Read the model definition and answer for the solid it produces. Units are mm, in the model's axes. A direction names the side the tool comes from. Coordinates: 2 decimals unless noted, no trailing zeros. Write each loop counter-clockwise with the first axis right and the second up, starting at its lowest first coordinate (ties: lowest second). Pieces come first, ordered by that corner, then holes.
Item 1: Section C-C (y = 10) is taken. Give the vertices of the cut face in (x, z) (3 decimals).
Item 2: Section B-B (x = 35) is taken. Give the vertices of the cut face in (y, z), then the cut area to 3 significant figures.
Item 3: A tool of negligible diameter and unlimited length cuts with its end or side. For faces 1 (the face through (-38.028, 7.919, 8.452)), 2 (the face through (36, 7, 30)), 3 (the face through (-37.5, 6.6, -0.1)), 4 (the face through (13.155, 6.409, -31.352)), from which of +Z, -Z, +X, -X, +Y, -Y can it reach the whole face along a straight path? Write none if from no direction.
Item 4: Determine the mould class of faces 5 (the face through (-36, 7, 30)), 6 (the face through (-9, 13, -33)), 7 (the face through (-31.352, 6.409, -13.155)) for opening direction Y: released by +Y, released by -Y, zero draft, split by the parting line, or undercut.
Item 5: Section D-D (z = -35) is taken. Give the vertices of the cut face in (x, y), then the cut area to 3 significant figures.
Item 6: Each of these flat-tipped pins is pushed along its axis until it touches: P1, Ø1.3, axis at y = 5.5, z = 30, coming from the -X side; P2, Ø3.5, axis at y = 6.5, z = 10, coming from the +X side; P3, Ø5, axis at y = 8, z = -23, coming from the +X side. Where does it stop, or does it pass through?
Item 7: Section A-A (z = 10) is taken. Give the vertices of the cut face in (x, y).
Item 8: Straight lines are drawn through the part: probe 1 along X at (y, z) = (10.5, 6.5); probe 2 along Y at (x, z) = (-37, 10); probe 3 along X at (y, z) = (7.75, 0). For each, find the intervals that lie inside material, in ascending order.
from build123d import *

# Parameters (mm, degrees)
SKETCH_1_R          = 34
EXTRUDE_1_DEPTH     = 13
SKETCH_2_R          = 2.5
CUT_EXTRUDE_1_DEPTH = 59.043087444
SKETCH_3_W          = 68
SKETCH_3_H          = 40
CUT_EXTRUDE_2_DEPTH = 59.043087444
SKETCH_4_R          = 2.1
CUT_EXTRUDE_3_DEPTH = 4


with BuildPart() as part:
    # 草图1 → 凸台-拉伸1 (new body)
    with BuildSketch(Plane(origin=(0, 0, 0), x_dir=(1, 0, 0), z_dir=(0, 1, 0))):
        with BuildLine():
            Line((-40, 0), (-40, -40))
            Line((-40, -40), (40, -40))
            Line((40, -40), (40, 0))
            ThreePointArc((40, 0), (0, 40), (-40, 0))
        make_face()
        with Locations(Location((0, 0, 0), (0, 0, 90))):
            Circle(SKETCH_1_R, mode=Mode.SUBTRACT)
    extrude(amount=EXTRUDE_1_DEPTH)

    # 草图2 → 切除-拉伸1 (cut, through all)
    with BuildSketch(Plane(origin=(0, 13, 0), x_dir=(1, 0, 0), z_dir=(0, 1, 0))):
        with Locations((0, 35)):
            Circle(SKETCH_2_R)
        with Locations((24.748737342, 24.748737342)):
            Circle(SKETCH_2_R)
        with Locations((35, 0)):
            Circle(SKETCH_2_R)
        with Locations((24.748737342, -24.748737342)):
            Circle(SKETCH_2_R)
        with Locations((0, -35)):
            Circle(SKETCH_2_R)
        with Locations((-24.748737342, -24.748737342)):
            Circle(SKETCH_2_R)
        with Locations((-35, 0)):
            Circle(SKETCH_2_R)
        with Locations((-24.748737342, 24.748737342)):
            Circle(SKETCH_2_R)
    extrude(amount=-CUT_EXTRUDE_1_DEPTH, mode=Mode.SUBTRACT)

    # 草图3 → 切除-拉伸2 (cut, through all)
    with BuildSketch(Plane(origin=(0, 13, 0), x_dir=(1, 0, 0), z_dir=(0, 1, 0))):
        with Locations((0, -20)):
            Rectangle(SKETCH_3_W, SKETCH_3_H)
    extrude(amount=-CUT_EXTRUDE_2_DEPTH, mode=Mode.SUBTRACT)

    # 草图4 → 切除-拉伸3 (cut)
    with BuildSketch(Plane.ZY.offset(40)):
        with Locations((10, 6.5)):
            Circle(SKETCH_4_R)
        with Locations((30, 6.5)):
            Circle(SKETCH_4_R)
    cut_extrude_3 = extrude(amount=-CUT_EXTRUDE_3_DEPTH, mode=Mode.SUBTRACT)

    # 镜向1: 切除-拉伸3 across plane
    add(cut_extrude_3.mirror(Plane.ZY), mode=Mode.SUBTRACT)


solid = part.part
Established:
1. outline: (-40, 0) arc R40 ccw to (40, 0) - (40, 40) - (34, 40) - (34, 2.291) arc R2.5 cw (long way) to (33.925, -2.257) arc R34 cw to (25.585, -22.393) arc R2.5 cw (long way) to (22.393, -25.585) arc R34 cw to (2.257, -33.925) arc R2.5 cw (long way) to (-2.257, -33.925) arc R34 cw to (-22.393, -25.585) arc R2.5 cw (long way) to (-25.585, -22.393) arc R34 cw to (-33.925, -2.257) arc R2.5 cw (long way) to (-34, 2.291) - (-34, 40) - (-40, 40) - close
2. outline: (0, -19.36) - (13, -19.36) - (13, -2.5) - (0, -2.5) - close; (0, 2.5) - (13, 2.5) - (13, 40) - (0, 40) - close
2. area: 707 mm2
3. face 1: -X
3. face 2: +X
3. face 3: +Y, -Y
3. face 4: +Z, +Y, -Y
4. face 5: undercut
4. face 6: released by +Y
4. face 7: zero draft
5. outline: (-19.36, 0) - (-2.5, 0) - (-2.5, 13) - (-19.36, 13) - close; (2.5, 0) - (19.36, 0) - (19.36, 13) - (2.5, 13) - close
5. area: 438 mm2
6. P1: stops at x = -36
6. P2: stops at x = 36
6. P3: stops at x = 34.35
7. outline: (-40, 0) - (-34, 0) - (-34, 13) - (-40, 13) - (-40, 8.6) - (-36, 8.6) - (-36, 4.4) - (-40, 4.4) - close; (34, 0) - (40, 0) - (40, 4.4) - (36, 4.4) - (36, 8.6) - (40, 8.6) - (40, 13) - (34, 13) - close
8. probe 1: x = -40 to -34, 34 to 40
8. probe 2: y = 0 to 4.4, 8.6 to 13
8. probe 3: x = -40 to -37.5, 37.5 to 40
